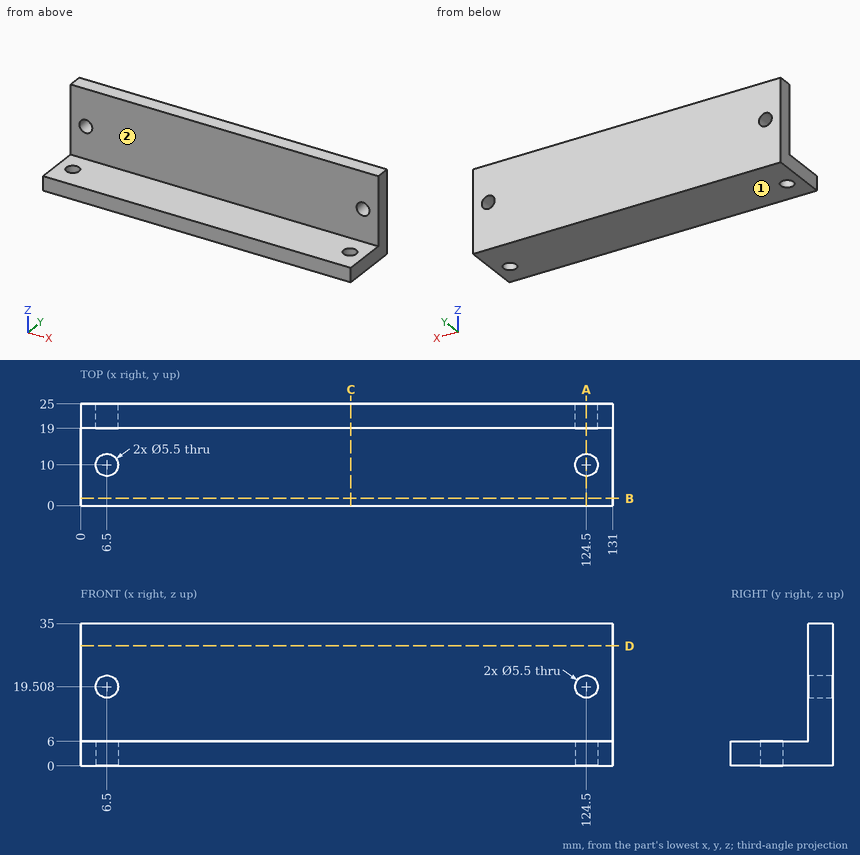
The figure shows three views and two pictorial views of one solid part (mm, origin at its lowest corner). Answer the questions. A direction names the side the tool comes from. Give positions to 0.01 mm unless a question says otherwise; leave off trailing zeros. Order: outer loops, then holes, each group sorted by start corner. A loop starts at its lowest first (then second) coordinate and runs counter-clockwise, first axis right, second up. Notation, with made-up numbers: (32, 3) -> (38, 3) arc R32 ccw to (38, 33) -> close; hole circle Ø2 at (-22, -24). An arc over 180 degrees is marked (long way). Answer as a JSON object with one key per item and string values. Group by question number.
Item 1: The part is cut by section B-B on y = 1.75. Write down the section's boundary in (x, z), and give its area (3 significant figures).
Item 2: Flat-ended cylindrical pins translate along their axes: pin 1 (6 mm diameter, centred on y = 17, z = 9.5, fed in from -X); pin 2 (7 mm diameter, centred on x = 6.5, z = 19.51, fed in from -Y); pin 3 (5.5 mm diameter, centred on x = 90, y = 10, fed in from +Z); pin 4 (3.5 mm diameter, centred on x = 124.5, y = 10, fed in from +Z). Find the tip coordinate at first contact, or state that the pin passes through.
Item 3: Consider L1, parallel to Y at x = 6.5, z = 4.55; L2, parallel to Z at x = 6.5, y = 23.3; L3, parallel to Z at x = 15.5, y = 15.75. Determine where each line is inside the solid, lowest interval first. Write a range as from..to.
Item 4: The part is cut by section A-A on x = 124.5. Write down the section's boundary in (y, z).
Item 5: A tool of negligible diameter and unlimited length cuts with its end or side. For the marked faces 1 and 2, from which of +Z, -Z, +X, -X, +Y, -Y can it reach the whole face along a straight path? Write none if from no direction.
Item 6: The part is cut by section C-C on x = 66.5. Write down the section's boundary in (y, z).
Item 7: The part is cut by section D-D on z = 29.5. Write down the section's boundary in (x, y), and give its area (3 significant figures).
Result set:
{
 "1": {"outline": "(0, 0) -> (131, 0) -> (131, 6) -> (0, 6) -> close", "area": "786 mm²"},
 "2": {"pin 1": "x = 0", "pin 2": "y = 19", "pin 3": "z = 6", "pin 4": "through"},
 "3": {"L1": "0..7.25, 12.75..25", "L2": "0..16.76, 22.26..35", "L3": "0..6"},
 "4": {"outline": "(0, 0) -> (7.25, 0) -> (7.25, 6) -> (0, 6) -> close; (12.75, 0) -> (25, 0) -> (25, 16.76) -> (19, 16.76) -> (19, 6) -> (12.75, 6) -> close; (19, 22.26) -> (25, 22.26) -> (25, 35) -> (19, 35) -> close"},
 "5": {"face 1": "-Z, +X, -X, +Y, -Y", "face 2": "+Z, +X, -X, -Y"},
 "6": {"outline": "(0, 0) -> (25, 0) -> (25, 35) -> (19, 35) -> (19, 6) -> (0, 6) -> close"},
 "7": {"outline": "(0, 19) -> (131, 19) -> (131, 25) -> (0, 25) -> close", "area": "786 mm²"}
}
